Build history of the part. All positions in model axes, mm. Round coordinates to 2 decimals unless told otherwise and drop trailing zeros. Write each loop counter-clockwise with the first axis right and the second up, starting at its lowest first coordinate (ties: lowest second). Pieces come first, ordered by that corner, then holes. Notation, with made-up numbers: (7.25, 74) -> (48.25, 74) arc R32 ccw to (48.25, 113) -> close; hole circle Ø9 at (76, 69). An arc over 180 degrees is marked (long way). Answer in a Markdown table with one row per item.
```python
from build123d import *

# Parameters (mm, degrees)
F0_W     = 38.1
F0_H     = 88.9
F1_DEPTH = 876.3


with BuildPart() as f1:
    # F0 (on Right) → F1 (new body)
    with BuildSketch(Plane.YZ):
        with BuildLine():
            ThreePointArc((25.4, 44.45), (23.540128, 48.940128), (19.05, 50.8))
            Line((19.05, 50.8), (-19.05, 50.8))
            ThreePointArc((-19.05, 50.8), (-23.540128, 48.940128), (-25.4, 44.45))
            Line((-25.4, 44.45), (-25.4, -44.45))
            ThreePointArc((-25.4, -44.45), (-23.540128, -48.940128), (-19.05, -50.8))
            Line((-19.05, -50.8), (19.05, -50.8))
            ThreePointArc((19.05, -50.8), (23.540128, -48.940128), (25.4, -44.45))
            Line((25.4, -44.45), (25.4, 44.45))
        make_face()
        Rectangle(F0_W, F0_H, mode=Mode.SUBTRACT)
    extrude(amount=-F1_DEPTH)


solid = f1.part
```
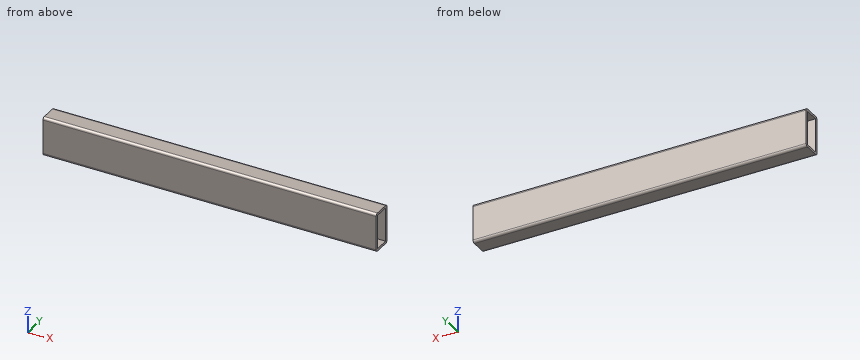
Q1. Saw through at C-C on x = -396. Write the cut outline in (y, z), plus the area to 3 significant figures.
A:
| item | result |
|---|---|
| outline | (-25.4, -44.45) arc R6.35 ccw to (-19.05, -50.8) -> (19.05, -50.8) arc R6.35 ccw to (25.4, -44.45) -> (25.4, 44.45) arc R6.35 ccw to (19.05, 50.8) -> (-19.05, 50.8) arc R6.35 ccw to (-25.4, 44.45) -> close; hole (-19.05, -44.45) -> (19.05, -44.45) -> (19.05, 44.45) -> (-19.05, 44.45) -> close |
| area | 1,740 mm² |
Q2. Saw through at A-A on z = -14. Write the cut outline in (x, y), plus the area to 3 significant figures.
A:
| item | result |
|---|---|
| outline | (-876.3, -25.4) -> (0, -25.4) -> (0, -19.05) -> (-876.3, -19.05) -> close; (-876.3, 19.05) -> (0, 19.05) -> (0, 25.4) -> (-876.3, 25.4) -> close |
| area | 11,100 mm² |
Q3. Saw through at B-B on y = -3. Write the cut outline in (x, z).
A:
| item | result |
|---|---|
| outline | (-876.3, -50.8) -> (0, -50.8) -> (0, -44.45) -> (-876.3, -44.45) -> close; (-876.3, 44.45) -> (0, 44.45) -> (0, 50.8) -> (-876.3, 50.8) -> close |
Q4. Wall check: line 1 (Y direction, x = -330.5, z = -42); line 2 (Z direction, x = -270.5, y = 7); line 3 (Z direction, x = -86, y = -20). Give the ranges that are in metal, low to high. Write a range as [from, to].
A:
| item | result |
|---|---|
| line 1 | [-25.4, -19.05], [19.05, 25.4] |
| line 2 | [-50.8, -44.45], [44.45, 50.8] |
| line 3 | [-50.73, 50.73] |
